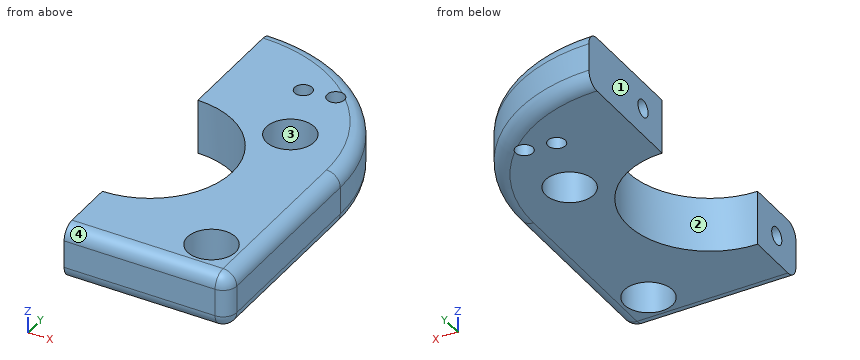
from build123d import *

# Parameters (mm, degrees)
SKETCH1_R                  = 5.55625
BOSS_EXTRUDE1_DEPTH        = 12.7
F_10_32_TAPPED_HOLE2_D     = 4.0386
F_10_32_TAPPED_HOLE3_D     = 4.0386
F_10_32_TAPPED_HOLE3_DEPTH = 16.002
F_10_32_TAPPED_HOLE3_TIP   = 1.213317848
FILLET1_R                  = 3.175


with BuildPart() as part:
    # Sketch1 → Boss-Extrude1 (new body)
    with BuildSketch(Plane.XY):
        with BuildLine():
            Line((-19.05, 0), (19.05, 0))
            Line((19.05, 0), (19.05, 44.45))
            ThreePointArc((19.05, 44.45), (7.890768363, 71.390768363), (-19.05, 82.55))
            Line((-19.05, 82.55), (-19.05, 53.34))
            ThreePointArc((-19.05, 53.34), (0, 34.29), (-19.05, 15.24))
            Line((-19.05, 15.24), (-19.05, 0))
        make_face()
        with Locations((9.525, 9.525)):
            Circle(SKETCH1_R, mode=Mode.SUBTRACT)
        with Locations((3.175, 51.914520005)):
            Circle(SKETCH1_R, mode=Mode.SUBTRACT)
    extrude(amount=BOSS_EXTRUDE1_DEPTH)

    # #10-32 Tapped Hole2 (through all)
    with Locations(Plane.XY.offset(12.7)):
        with Locations((-2.630812741, 67.096934822), (4.277109037, 68.131749636)):
            Hole(F_10_32_TAPPED_HOLE2_D / 2)

    # #10-32 Tapped Hole3
    with Locations(Plane.ZY.offset(19.05)):
        with Locations((6.35, 7.62), (6.35, 60.96)):
            Hole(F_10_32_TAPPED_HOLE3_D / 2, depth=F_10_32_TAPPED_HOLE3_DEPTH)
            with Locations((0, 0, -(F_10_32_TAPPED_HOLE3_DEPTH + F_10_32_TAPPED_HOLE3_TIP / 2))):  # 118° drill point
                Cone(0, F_10_32_TAPPED_HOLE3_D / 2, F_10_32_TAPPED_HOLE3_TIP, mode=Mode.SUBTRACT)

    # Fillet1
    # the kernel refuses this fillet: 3.175 mm, written as the material it takes off along each edge
    with BuildSketch(Plane(origin=(15.875, 3.175, 9.525), x_dir=(0, -1, 0), z_dir=(0, 0, 1))) as fillet1_piece_1_section:
        Polygon((0, 0), (FILLET1_R * 1.02, 0), (FILLET1_R * 1.02, FILLET1_R * 1.02), (0, FILLET1_R * 1.02), align=None)
    fillet1_piece_1 = extrude(amount=FILLET1_R * 1.02, mode=Mode.PRIVATE)
    fillet1_piece_1 = fillet1_piece_1 - Plane(origin=(15.875, 3.175, 9.525), x_dir=(-0.7071067811865476, 0.7071067811865475, 0), z_dir=(0, 0, 1)) * Sphere(FILLET1_R, mode=Mode.PRIVATE)
    add(fillet1_piece_1, mode=Mode.SUBTRACT)
    with BuildSketch(Plane(origin=(15.875, 3.175, 3.175), x_dir=(0, -1, 0), z_dir=(0, 0, -1))) as fillet1_piece_2_section:
        Polygon((0, 0), (FILLET1_R * 1.02, 0), (FILLET1_R * 1.02, -FILLET1_R * 1.02), (0, -FILLET1_R * 1.02), align=None)
    fillet1_piece_2 = extrude(amount=FILLET1_R * 1.02, mode=Mode.PRIVATE)
    fillet1_piece_2 = fillet1_piece_2 - Plane(origin=(15.875, 3.175, 3.175), x_dir=(-0.7071067811865476, 0.7071067811865475, 0), z_dir=(0, 0, -1)) * Sphere(FILLET1_R, mode=Mode.PRIVATE)
    add(fillet1_piece_2, mode=Mode.SUBTRACT)
    with BuildSketch(Plane(origin=(19.05, 3.175, 12.7), x_dir=(-1, 0, 0), z_dir=(0, 1, 0))) as fillet1_piece_3:
        with BuildLine():
            CenterArc((FILLET1_R, -FILLET1_R), FILLET1_R, 90, 90)
            Line((0, -FILLET1_R), (-FILLET1_R * 0.02, -FILLET1_R))
            Line((-FILLET1_R * 0.02, -FILLET1_R), (-FILLET1_R * 0.02, FILLET1_R * 0.02))
            Line((-FILLET1_R * 0.02, FILLET1_R * 0.02), (FILLET1_R, FILLET1_R * 0.02))
            Line((FILLET1_R, FILLET1_R * 0.02), (FILLET1_R, 0))
        make_face()
    extrude(amount=41.275, mode=Mode.SUBTRACT)
    with BuildSketch(Plane(origin=(19.05, 0, 3.175), x_dir=(-1, 0, 0), z_dir=(0, 0, 1))) as fillet1_piece_4:
        with BuildLine():
            CenterArc((FILLET1_R, -FILLET1_R), FILLET1_R, 90, 90)
            Line((0, -FILLET1_R), (-FILLET1_R * 0.02, -FILLET1_R))
            Line((-FILLET1_R * 0.02, -FILLET1_R), (-FILLET1_R * 0.02, FILLET1_R * 0.02))
            Line((-FILLET1_R * 0.02, FILLET1_R * 0.02), (FILLET1_R, FILLET1_R * 0.02))
            Line((FILLET1_R, FILLET1_R * 0.02), (FILLET1_R, 0))
        make_face()
    extrude(amount=6.35, mode=Mode.SUBTRACT)
    with BuildSketch(Plane(origin=(-19.05, 44.45, 12.7), x_dir=(1, 0, 0), z_dir=(0, -1, 0))) as fillet1_piece_5:
        with BuildLine():
            CenterArc((38.1 - FILLET1_R, -FILLET1_R), FILLET1_R, 0, 90)
            Line((38.1, -FILLET1_R), (38.1 + FILLET1_R * 0.02, -FILLET1_R))
            Line((38.1 + FILLET1_R * 0.02, -FILLET1_R), (38.1 + FILLET1_R * 0.02, FILLET1_R * 0.02))
            Line((38.1 + FILLET1_R * 0.02, FILLET1_R * 0.02), (38.1 - FILLET1_R, FILLET1_R * 0.02))
            Line((38.1 - FILLET1_R, FILLET1_R * 0.02), (38.1 - FILLET1_R, 0))
        make_face()
    revolve(axis=Axis((-19.05, 44.45, 12.7), (0, 0, 1)), revolution_arc=90, mode=Mode.SUBTRACT)
    with BuildSketch(Plane(origin=(-19.05, 44.45, 0), x_dir=(1, 0, 0), z_dir=(0, -1, 0))) as fillet1_piece_6:
        with BuildLine():
            CenterArc((38.1 - FILLET1_R, FILLET1_R), FILLET1_R, 270, 90)
            Line((38.1, FILLET1_R), (38.1 + FILLET1_R * 0.02, FILLET1_R))
            Line((38.1 + FILLET1_R * 0.02, FILLET1_R), (38.1 + FILLET1_R * 0.02, -FILLET1_R * 0.02))
            Line((38.1 + FILLET1_R * 0.02, -FILLET1_R * 0.02), (38.1 - FILLET1_R, -FILLET1_R * 0.02))
            Line((38.1 - FILLET1_R, -FILLET1_R * 0.02), (38.1 - FILLET1_R, 0))
        make_face()
    revolve(axis=Axis((-19.05, 44.45, 0), (0, 0, 1)), revolution_arc=90, mode=Mode.SUBTRACT)
    with BuildSketch(Plane(origin=(-19.05, 0, 12.7), x_dir=(0, 1, 0), z_dir=(1, 0, 0))) as fillet1_piece_7:
        with BuildLine():
            CenterArc((FILLET1_R, -FILLET1_R), FILLET1_R, 90, 90)
            Line((0, -FILLET1_R), (-FILLET1_R * 0.02, -FILLET1_R))
            Line((-FILLET1_R * 0.02, -FILLET1_R), (-FILLET1_R * 0.02, FILLET1_R * 0.02))
            Line((-FILLET1_R * 0.02, FILLET1_R * 0.02), (FILLET1_R, FILLET1_R * 0.02))
            Line((FILLET1_R, FILLET1_R * 0.02), (FILLET1_R, 0))
        make_face()
    extrude(amount=34.925, mode=Mode.SUBTRACT)
    with BuildSketch(Plane(origin=(19.05, 3.175, 0), x_dir=(-1, 0, 0), z_dir=(0, 1, 0))) as fillet1_piece_8:
        with BuildLine():
            CenterArc((FILLET1_R, FILLET1_R), FILLET1_R, 180, 90)
            Line((0, FILLET1_R), (-FILLET1_R * 0.02, FILLET1_R))
            Line((-FILLET1_R * 0.02, FILLET1_R), (-FILLET1_R * 0.02, -FILLET1_R * 0.02))
            Line((-FILLET1_R * 0.02, -FILLET1_R * 0.02), (FILLET1_R, -FILLET1_R * 0.02))
            Line((FILLET1_R, -FILLET1_R * 0.02), (FILLET1_R, 0))
        make_face()
    extrude(amount=41.275, mode=Mode.SUBTRACT)
    with BuildSketch(Plane(origin=(-19.05, 0, 0), x_dir=(0, 1, 0), z_dir=(1, 0, 0))) as fillet1_piece_9:
        with BuildLine():
            CenterArc((FILLET1_R, FILLET1_R), FILLET1_R, 180, 90)
            Line((0, FILLET1_R), (-FILLET1_R * 0.02, FILLET1_R))
            Line((-FILLET1_R * 0.02, FILLET1_R), (-FILLET1_R * 0.02, -FILLET1_R * 0.02))
            Line((-FILLET1_R * 0.02, -FILLET1_R * 0.02), (FILLET1_R, -FILLET1_R * 0.02))
            Line((FILLET1_R, -FILLET1_R * 0.02), (FILLET1_R, 0))
        make_face()
    extrude(amount=34.925, mode=Mode.SUBTRACT)


solid = part.part
Verification items for the finished model (mm, model axes). Face numbers are marked on the shaded views. Give positions to 0.01 mm unless a question says otherwise; leave off trailing zeros. Write each loop counter-clockwise with the first axis right and the second up, starting at its lowest first coordinate (ties: lowest second). Pieces come first, ordered by that corner, then holes. Notation, with made-up numbers: M 10,83 L 38,83 A10 cw 38,102 Z; hole C 29,86.25 d9. An arc over 180 degrees is marked long. Write item = value, one per line.
(1) Material ranges on line 1 (Z direction, x = -7.5, y = 7.62); line 2 (Y direction, x = -15, z = 6.35); line 3 (X direction, y = 67, z = 9), recorded low to high.
Found:
line_1 = 0 to 4.33, 8.37 to 12.7
line_2 = 0 to 5.6, 9.64 to 15.68, 52.9 to 58.94, 62.98 to 82.33
line_3 = -19.05 to -4.65, -0.61 to 2.6, 5.95 to 11.66
(2) Draft check along Y on the marked faces 1, 2, 3 and 4. Enter one of: released by +Y, released by -Y, zero draft, split by the parting line, or undercut.
Found:
face_1 = zero draft
face_2 = undercut
face_3 = undercut
face_4 = released by -Y
(3) Sectioned sample at A-A (y = 34.29). Record the cut outline in (x, z) (3 decimals).
Found:
outline = M 0,0 L 15.875,0 A3.175 ccw 19.05,3.175 L 19.05,9.525 A3.175 ccw 15.875,12.7 L 0,12.7 Z
(4) Sectioned sample at B-B (z = 11.25). Give the number of separate pieces and of enclosed holes in the cut face, then the cut area to 3 significant figures.
Found:
separate_pieces = 1
enclosed_holes = 4
area = 1,970 mm2
(5) Go/stop test with flat-tipped pins: pin 1 Ø5 at (x, z) = (-14.5, 5) entering from +Y; pin 2 Ø4 at (y, z) = (67.5, 5.5) entering from +X; pin 3 Ø6 at (y, z) = (42.5, 2) entering from -X; pin 4 Ø10 at (x, y) = (3.18, 51.91) entering from -Z. Record where each tip stops, or that it passes through.
Found:
pin_1 = 82.49
pin_2 = 12.71
pin_3 = -3.65
pin_4 = through
